```python
from build123d import *

# Parameters (mm, degrees)
BOSS_EXTRUDE1_DEPTH = 22.25
FILLET1_R           = 5
CUT_EXTRUDE1_REACH  = 44.254
SKETCH6_R           = 3.6
CUT_EXTRUDE2_REACH  = 44.254
SKETCH7_R           = 3.6


with BuildPart() as part:
    # Sketch2 → Boss-Extrude1 (new body)
    with BuildSketch(Plane.XY):
        Polygon((0, 25.4), (0, 0), (25.4, 0), (25.4, 4.75), (4.75, 4.75), (4.75, 25.4), align=None)
    extrude(amount=BOSS_EXTRUDE1_DEPTH)

    # Fillet1
    # the kernel refuses this fillet: 5 mm, written as the material it takes off along each edge
    with BuildSketch(Plane(origin=(4.75, 25.4, -12.484365222), x_dir=(0, -1, 0), z_dir=(0, 0, 1))) as fillet1_piece_1:
        with BuildLine():
            CenterArc((4.993746089, -5), FILLET1_R, 90, 87.134016017)
            Line((0, -4.75), (-0.099874922, -4.745))
            ThreePointArc((-0.099874922, -4.745), (-0.1, -2.375), (-0.1, 0))
            Line((-0.1, 0), (0, 0.1))
            Line((0, 0.1), (4.993746089, 0.1))
            Line((4.993746089, 0.1), (4.993746089, 0))
        make_face()
    extrude(amount=47.218730444, mode=Mode.SUBTRACT)
    with BuildSketch(Plane(origin=(25.4, 4.75, -12.484365222), x_dir=(0, -1, 0), z_dir=(0, 0, 1))) as fillet1_piece_2:
        with BuildLine():
            CenterArc((5, -4.993746089), FILLET1_R, 92.865983983, 87.134016017)
            Line((0, -4.993746089), (-0.1, -4.993746089))
            Line((-0.1, -4.993746089), (-0.1, 0))
            Line((-0.1, 0), (0, 0.1))
            ThreePointArc((0, 0.1), (2.375, 0.1), (4.745, 0.099874922))
            Line((4.745, 0.099874922), (4.75, 0))
        make_face()
    extrude(amount=47.218730444, mode=Mode.SUBTRACT)

    # Sketch6 → Cut-Extrude1 (cut, up to next)
    with BuildSketch(Plane.XZ, mode=Mode.PRIVATE) as cut_extrude1_sk1:
        with Locations(Location((12.7, 11.125, 0), (0, 0, 270))):
            Circle(SKETCH6_R)
    cut_extrude1_tool1 = extrude(cut_extrude1_sk1.sketch, amount=-CUT_EXTRUDE1_REACH, mode=Mode.PRIVATE) & part.part
    add(cut_extrude1_tool1.solids().sort_by_distance((12.7, 0, 11.125))[0], mode=Mode.SUBTRACT)

    # Sketch7 → Cut-Extrude2 (cut, up to next)
    with BuildSketch(Plane.ZY, mode=Mode.PRIVATE) as cut_extrude2_sk1:
        with Locations((11.125, 12.7)):
            Circle(SKETCH7_R)
    cut_extrude2_tool1 = extrude(cut_extrude2_sk1.sketch, amount=-CUT_EXTRUDE2_REACH, mode=Mode.PRIVATE) & part.part
    add(cut_extrude2_tool1.solids().sort_by_distance((0, 12.7, 11.125))[0], mode=Mode.SUBTRACT)


solid = part.part
```
The model under review builds one solid part; all positions refer to its coordinate system, in mm. A direction names the side the tool comes from. Round coordinates to 2 decimals unless told otherwise and drop trailing zeros. Loops run counter-clockwise (first coordinate to the right, second up) from the corner with the lowest first, then second, coordinate; pieces in that order, holes last. Notation, with made-up numbers: M 0.5,-20.75 L 18.5,-20.75 A10 cw 18.5,-16.75 Z; hole C 59.5,47.5 d7. An arc over 180 degrees is marked long. Put each result on its own line as item: value.
Q1. To check wall thickness, follow L1, parallel to Y at x = 11.75, z = 6.5; L2, parallel to Z at x = 4, y = 15. State the ranges of each line that lie inside material, in increasing order.
Result set:
L1: y = 0 to 4.75
L2: z = 0 to 8.36, 13.89 to 22.25
Q2. Machinability: for faces 5 (the flat face through (4.75, 9, 8)), 6 (the flat face through (10, 0, 8)), which of the approach directions +Z, -Z, +X, -X, +Y, -Y give a long, thin tool a straight path to every point of the face, cutting with its end or side? Answer none if there is none.
Result set:
face 5: +Z, -Z, +X, +Y
face 6: +Z, -Z, +X, -X, -Y
Q3. Consider section C-C, the plane z = 13. Give the boundary of the cut face in (x, y), then the cut area to 3 significant figures.
Result set:
outline: M 0,0 L 9.63,0 L 9.63,4.75 L 4.75,4.75 L 4.75,9.63 L 0,9.63 Z; M 0,15.77 L 4.75,15.77 L 4.75,20.41 A5 ccw 0,25.4 Z; M 15.77,0 L 25.4,0 A5 ccw 20.41,4.75 L 15.77,4.75 Z
area: 150 mm²
Q4. Mouldability with a two-part tool opening along Z and no side actions: class faces 1 (the cylindrical face through (23.891, 3.336, 10.969)), 2 (the cylindrical face through (11.32, 2.34, 7.8)), 3 (the flat face through (4, 7, 22.25)), 4 (the cylindrical face through (2.34, 11.32, 14.45)) as released by +Z, released by -Z, zero draft, split by the parting line, or undercut.
Result set:
face 1: zero draft
face 2: undercut
face 3: released by +Z
face 4: undercut
Q5. Consider section D-D, the plane z = 1.75. Give the boundary of the cut face in (x, y).
Result set:
outline: M 0,0 L 25.4,0 A5 ccw 20.41,4.75 L 4.75,4.75 L 4.75,20.41 A5 ccw 0,25.4 Z
Q6. For pin 1 (11.5 mm diameter, centred on y = 12.7, z = 11.125, fed in from +X); pin 2 (3 mm diameter, centred on y = 5, z = 10, fed in from +X); pin 3 (12.5 mm diameter, centred on x = 8.5, z = 8.5, fed in from +Y), all flat-tipped, find the tip position at first contact; note any pin that passes through.
Result set:
pin 1: stops at x = 4.75
pin 2: stops at x = 23.71
pin 3: stops at y = 24.74
Q7. Consider section A-A, the plane y = 12.7. Give the boundary of the cut face in (x, z) (3 decimals), then the cut area to 3 significant figures.
Result set:
outline: M 0,0 L 4.75,0 L 4.75,7.525 L 0,7.525 Z; M 0,14.725 L 4.75,14.725 L 4.75,22.25 L 0,22.25 Z
area: 71.5 mm²
